```python
from build123d import *

# Parameters (mm, degrees)
F0_W     = 568.325
F0_H     = 149.225
F1_DEPTH = 908.05
F2_T     = -3.175
F3_W     = 568.325
F3_H     = 36.4719758213
F4_DEPTH = 25.4
F5_T     = -3.175


# Not quite as in the source:
# - a shell that OpenCascade refuses in one call is made with other operations: the cavity is built on its own and cut out


with BuildPart() as f1:
    # F0 (on Front) → F1 (new body)
    with BuildSketch(Plane.XZ):
        Rectangle(F0_W, F0_H)
    extrude(amount=F1_DEPTH)

    # F2
    f2_openings = [f1.faces().sort_by_distance(p)[0] for p in [
        (0, -454.025, 74.6125),
    ]]
    offset(amount=F2_T, openings=f2_openings)

    # F3 (on face) → F4 (join)
    with BuildSketch(Plane.XZ.offset(908.05)):
        with Locations((0, 56.3765120894)):
            Rectangle(F3_W, F3_H)
    extrude(amount=F4_DEPTH)

    # F5: a shell. OpenCascade refuses it in one call, so the cavity is built on its own and cut out:
    # the body offset inwards by the wall thickness, plus a prism from it out through each open face.
    f5_core = offset(f1.part, amount=F5_T, kind=Kind.INTERSECTION, mode=Mode.PRIVATE)
    f5_exits = [f5_core.faces().sort_by_distance(p)[0] for p in [
        (0, -919.1625, 41.315524),
    ]]
    add(f5_core, mode=Mode.SUBTRACT)
    extrude(f5_exits, amount=-F5_T, mode=Mode.SUBTRACT)


solid = f1.part
```
Geometry check sheet. Reference: the model listing, model coordinates, mm. A direction names the side the tool comes from. Give positions to 0.01 mm unless a question says otherwise; leave off trailing zeros. Write each loop counter-clockwise with the first axis right and the second up, starting at its lowest first coordinate (ties: lowest second). Pieces come first, ordered by that corner, then holes.
1) Gauge pin test, flat ends, axial feed: pin 1 (3 mm diameter, centred on x = -51, z = -15, fed in from -Y); pin 2 (1.5 mm diameter, centred on x = 149, y = -415.5, fed in from +Z). Record the tip position at first contact, or that the pin passes through.
2) Material ranges on L1, parallel to Y at x = 7.5, z = 55 (3 decimals); L2, parallel to X at y = -520, z = 23; L3, parallel to Y at x = -109, z = 38 (3 decimals), recorded low to high.
3) Release check for a two-part mould opening along Y. For faces 6 (the flat face through (-4, -904.875, 3)), 7 (the flat face through (-1, -914, 74.613)), 8 (the flat face through (280.988, -919, 55)), 9 (the flat face through (-4, -933.45, 57)) record: pulls with the +Y half, pulls with the -Y half, needs draft (parallel to the pull), parting line crosses it, or undercut.
4) Access from +Z, -Z, +X, -X, +Y, -Y to the whole of each face (thin tool, end or side, straight path). Record for faces 1 (the flat face through (4, -930.275, 55)), 2 (the flat face through (-4, -448, -74.612)), 3 (the flat face through (-1, -932, 38.141)), 4 (the flat face through (284.162, -460, -1)), 5 (the flat face through (-280.988, -448, 1)).
5) Section check A-A, the plane z = 48.5. State how many separate pieces and enclosed holes the cut face has, and give its area (3 significant figures).
6) Section check D-D, the plane y = -280. Record the boundary of the cut face in (x, z).
Computed:
1. pin 1: stops at y = -908.05
1. pin 2: stops at z = -71.44
2. L1: y = -933.45 to -930.275, -908.05 to -904.875, -3.175 to 0
2. L2: x = -284.16 to -280.99, 280.99 to 284.16
2. L3: y = -908.05 to -904.875, -3.175 to 0
3. face 6: undercut
3. face 7: needs draft
3. face 8: undercut
3. face 9: pulls with the -Y half
4. face 1: -Z
4. face 2: -Z, +X, -X, +Y, -Y
4. face 3: -Z, +X, -X, -Y
4. face 4: +Z, -Z, +X, +Y, -Y
4. face 5: +Z
5. separate pieces: 1
5. enclosed holes: 2
5. area: 11,300 mm2
6. outline: (-284.16, -74.61) - (284.16, -74.61) - (284.16, 74.61) - (280.99, 74.61) - (280.99, -71.44) - (-280.99, -71.44) - (-280.99, 74.61) - (-284.16, 74.61) - close
